Source: three-view drawing plus pictorial views. Frame: mm from the lowest corner of the part. Give positions to 0.01 mm unless a question says otherwise; leave off trailing zeros. Loops run counter-clockwise (first coordinate to the right, second up) from the corner with the lowest first, then second, coordinate; pieces in that order, holes last. Notation, with made-up numbers: (87, -26) - (97, -26) arc R12 cw to (97, -15) - close; hole circle Ø4 at (52, 49). An arc over 180 degrees is marked (long way). Write each question's results on one line, items separated by ' | '. Start each with the question number.
(1) Cut plane A-A on x = 0.9. Return the cut outline in (y, z) (1 decimal).
(2) Cut plane B-B on z = 2.1. Return the cut outline in (x, y) (1 decimal).
(3) Cut plane C-C on y = 5.25. Return the cut outline in (x, z) (1 decimal).
(4) Material intervals for line 1 along Z through (x, y) = (1.4, 7.5) (1 decimal); line 2 along Y through (x, z) = (0.7, 1.15) (1 decimal), sorted ascending. Write a range as [from, to].
(5) Contact query for flat-ended pins moving along their axis: pin 1 (0.6 mm diameter, centred on x = 1.5, y = 8.5, fed in from +Z); pin 2 (0.6 mm diameter, centred on x = 1.5, y = 2, fed in from -Z); pin 3 (0.6 mm diameter, centred on y = 2, z = 1.5, fed in from -X); pin 4 (0.6 mm diameter, centred on x = 1, z = 1.5, fed in from +Y). Output: stop coordinate, or through.
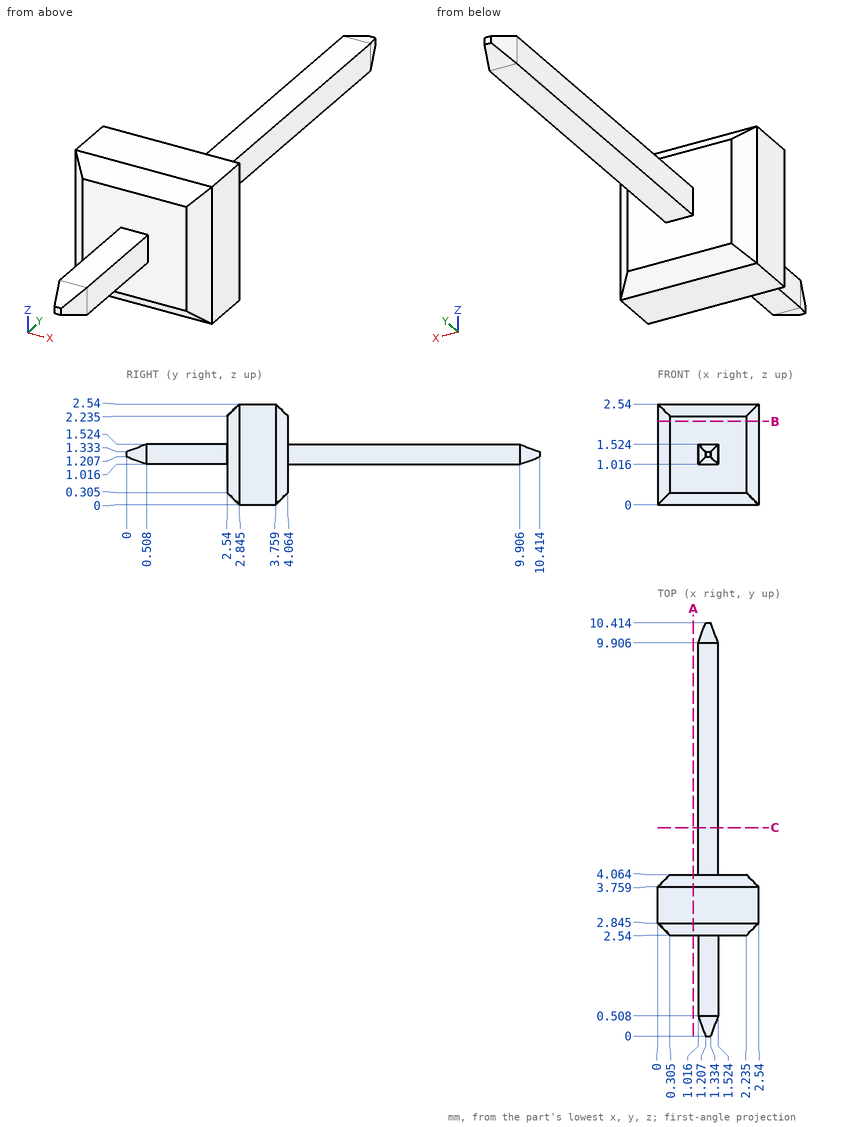
Ans:
1) outline: (2.5, 0.3) - (2.8, 0) - (3.8, 0) - (4.1, 0.3) - (4.1, 2.2) - (3.8, 2.5) - (2.8, 2.5) - (2.5, 2.2) - close
2) outline: (0, 2.8) - (0.3, 2.5) - (2.2, 2.5) - (2.5, 2.8) - (2.5, 3.8) - (2.2, 4.1) - (0.3, 4.1) - (0, 3.8) - close
3) outline: (1, 1) - (1.5, 1) - (1.5, 1.5) - (1, 1.5) - close
4) line 1: [1, 1.5] | line 2: [2.5, 4.1]
5) pin 1: z = 1.52 | pin 2: z = 1.02 | pin 3: x = 1.02 | pin 4: y = 10.41
